Input: part model. Units: mm. Frame: model coordinates. A direction names the side the tool comes from. Round coordinates to 2 decimals unless told otherwise and drop trailing zeros. Loops run counter-clockwise (first coordinate to the right, second up) from the corner with the lowest first, then second, coordinate; pieces in that order, holes last.
1) Section D-D, the plane y = -22.5. Return loops of the section in (x, z), and give its area (3 significant figures).
2) Ray query, line 1 along X through (y, z) = (27, 0.55); line 2 along Y through (x, z) = (49, 0.75) (3 decimals); line 3 along Y through (x, z) = (10.5, 0.5). Return the intervals inside material, ascending.
3) Access query for faces 1 (the face through (26.94, 31.3, 0.78)), 2 (the face through (26.742, -37.615, 0.783)), 3 (the face through (-7.924, -11.766, 0.783)). Directions: +Z, -Z, +X, -X, +Y, -Y. A direction counts if a zero-diameter tool reaches every point of the face in a straight line with its end or side. Return the directions, or none.
4) Section A-A, the plane x = 25. Return loops of the section in (y, z).
5) Draft query along X for faces 4 (the face through (54.83, -43.89, 0.78)), 5 (the face through (-7.51, -29.71, 0.78)), 6 (the face through (2, -3, 1.588)). Return one class per face: pulls with the +X half, pulls with the -X half, needs draft (parallel to the pull), parting line crosses it, or undercut.
6) Section C-C, the plane z = 0.35. State how many separate pieces and enclosed holes the cut face has, and give its area (3 significant figures).
7) First-contact query: pin 1 (0.8 mm diameter, centred on x = 2, z = 0.5, fed in from -Y); pin 2 (0.5 mm diameter, centred on y = -40.5, z = 0.5, fed in from -X). Flat tips, straight axial feed; report the tip coordinate or a pass-through.
8) Section B-B, the plane x = -19. Return loops of the section in (y, z).
from build123d import *

# Parameters (mm, degrees)
F0_R     = 0.993004
F0_R_2   = 1.444011
F1_DEPTH = 1.5875


with BuildPart() as f1:
    # F0 (on Top) → F1 (new body)
    with BuildSketch(Plane.XY):
        with BuildLine():
            Line((-14.723098, 26.865108), (-29.863264, 35.613344))
            ThreePointArc((-29.863264, 35.613344), (-50.45729, 37.191393), (-38.937857, 20.047683))
            Line((-38.937857, 20.047683), (-12.721558, 4.9235))
            Line((-12.721558, 4.9235), (-11.685765, 4.128267))
            Line((-11.685765, 4.128267), (-10.891915, 3.094106))
            Line((-10.891915, 3.094106), (-10.393018, 1.886993))
            Line((-10.393018, 1.886993), (-10.222391, 0.594116))
            Line((-10.222391, 0.594116), (-10.220915, -7.038907))
            Line((-10.220915, -7.038907), (-10.393611, -8.33664))
            Line((-10.393611, -8.33664), (-10.893255, -9.537127))
            Line((-10.893255, -9.537127), (-11.691344, -10.573302))
            Line((-11.691344, -10.573302), (-12.744763, -11.375137))
            Line((-12.744763, -11.375137), (-38.796974, -26.421059))
            Line((-38.796974, -26.421059), (-38.877102, -26.468848))
            ThreePointArc((-38.877102, -26.468848), (-50.486605, -43.553232), (-29.883725, -42.077399))
            Line((-29.883725, -42.077399), (-14.723923, -33.307276))
            Line((-14.723923, -33.307276), (-13.889479, -32.979281))
            Line((-13.889479, -32.979281), (-12.998538, -32.911762))
            Line((-12.998538, -32.911762), (-12.125839, -33.111285))
            Line((-12.125839, -33.111285), (-11.353738, -33.556437))
            Line((-11.353738, -33.556437), (-10.745112, -34.212011))
            Line((-10.745112, -34.212011), (-10.356967, -35.016805))
            Line((-10.356967, -35.016805), (-10.221996, -35.901241))
            Line((-10.221996, -35.901241), (-10.221996, -46.300355))
            Line((-10.221996, -46.300355), (-10.074989, -47.230888))
            Line((-10.074989, -47.230888), (-9.656024, -48.045732))
            Line((-9.656024, -48.045732), (-8.990064, -48.723656))
            Line((-8.990064, -48.723656), (-8.144654, -49.150351))
            Line((-8.144654, -49.150351), (-7.219487, -49.297899))
            Line((-7.219487, -49.297899), (11.685274, -49.296624))
            Line((11.685274, -49.296624), (12.637615, -49.147114))
            Line((12.637615, -49.147114), (13.504221, -48.70079))
            Line((13.504221, -48.70079), (14.18661, -48.018399))
            Line((14.18661, -48.018399), (14.627374, -47.158636))
            Line((14.627374, -47.158636), (14.775819, -46.2091))
            Line((14.775819, -46.2091), (14.778971, -35.906233))
            Line((14.778971, -35.906233), (14.910567, -35.024933))
            Line((14.910567, -35.024933), (15.297383, -34.217406))
            Line((15.297383, -34.217406), (15.907513, -33.557428))
            Line((15.907513, -33.557428), (16.67915, -33.11279))
            Line((16.67915, -33.11279), (17.548487, -32.913399))
            Line((17.548487, -32.913399), (18.445739, -32.979199))
            Line((18.445739, -32.979199), (19.277777, -33.305883))
            Line((19.277777, -33.305883), (34.417649, -42.047282))
            ThreePointArc((34.417649, -42.047282), (55.015649, -43.582376), (43.457552, -26.463833))
            Line((43.457552, -26.463833), (17.281802, -11.366066))
            Line((17.281802, -11.366066), (16.244157, -10.573521))
            Line((16.244157, -10.573521), (15.449484, -9.535828))
            Line((15.449484, -9.535828), (14.94993, -8.331098))
            Line((14.94993, -8.331098), (14.780158, -7.041344))
            Line((14.780158, -7.041344), (14.780158, 0.595206))
            Line((14.780158, 0.595206), (14.94993, 1.885977))
            Line((14.94993, 1.885977), (15.448278, 3.091799))
            Line((15.448278, 3.091799), (16.244157, 4.133809))
            Line((16.244157, 4.133809), (17.277955, 4.923416))
            Line((17.277955, 4.923416), (43.350993, 19.979317))
            ThreePointArc((43.350993, 19.979317), (54.979423, 37.050162), (34.375281, 35.599827))
            Line((34.375281, 35.599827), (19.284697, 26.87011))
            Line((19.284697, 26.87011), (18.450038, 26.540194))
            Line((18.450038, 26.540194), (17.539247, 26.472519))
            Line((17.539247, 26.472519), (16.68203, 26.667085))
            Line((16.68203, 26.667085), (15.906996, 27.120017))
            Line((15.906996, 27.120017), (15.300046, 27.770561))
            Line((15.300046, 27.770561), (14.911061, 28.57871))
            Line((14.911061, 28.57871), (14.778835, 29.453185))
            Line((14.778835, 29.453185), (14.778835, 39.838884))
            Line((14.778835, 39.838884), (14.635858, 40.771108))
            Line((14.635858, 40.771108), (14.205475, 41.613926))
            Line((14.205475, 41.613926), (13.539729, 42.286281))
            Line((13.539729, 42.286281), (12.708107, 42.70209))
            Line((12.708107, 42.70209), (11.775819, 42.852354))
            Line((11.775819, 42.852354), (9.028588, 42.849436))
            Line((9.028588, 42.849436), (8.248972, 42.750109))
            Line((8.248972, 42.750109), (7.521199, 42.450108))
            Line((7.521199, 42.450108), (6.899957, 41.975875))
            Line((6.899957, 41.975875), (6.155663, 41.238896))
            Line((6.155663, 41.238896), (5.542562, 40.758778))
            Line((5.542562, 40.758778), (4.811539, 40.46033))
            Line((4.811539, 40.46033), (4.057043, 40.356379))
            Line((4.057043, 40.356379), (0.515512, 40.356379))
            Line((0.515512, 40.356379), (-0.251471, 40.45441))
            Line((-0.251471, 40.45441), (-0.987362, 40.755984))
            Line((-0.987362, 40.755984), (-1.601019, 41.228801))
            Line((-1.601019, 41.228801), (-2.333428, 41.96848))
            Line((-2.333428, 41.96848), (-2.958887, 42.448372))
            Line((-2.958887, 42.448372), (-3.688263, 42.751611))
            Line((-3.688263, 42.751611), (-4.465904, 42.852182))
            Line((-4.465904, 42.852182), (-7.223364, 42.850204))
            Line((-7.223364, 42.850204), (-8.143452, 42.702295))
            Line((-8.143452, 42.702295), (-8.975075, 42.283129))
            Line((-8.975075, 42.283129), (-9.64701, 41.617799))
            Line((-9.64701, 41.617799), (-10.078163, 40.777281))
            Line((-10.078163, 40.777281), (-10.221545, 39.848268))
            Line((-10.221545, 39.848268), (-10.221545, 29.468842))
            Line((-10.221545, 29.468842), (-10.356562, 28.594707))
            Line((-10.356562, 28.594707), (-10.741985, 27.769495))
            Line((-10.741985, 27.769495), (-11.349, 27.124543))
            Line((-11.349, 27.124543), (-12.121995, 26.674023))
            Line((-12.121995, 26.674023), (-12.989837, 26.475296))
            Line((-12.989837, 26.475296), (-13.889652, 26.536117))
            Line((-13.889652, 26.536117), (-14.723098, 26.865108))
        make_face()
        with Locations((-41.662121, -42.13991)):
            Circle(F0_R, mode=Mode.SUBTRACT)
        with Locations((-36.148938, -38.95656)):
            Circle(F0_R, mode=Mode.SUBTRACT)
        with Locations((-44.843597, -36.637466)):
            Circle(F0_R, mode=Mode.SUBTRACT)
        with Locations((-39.334769, -33.438058)):
            Circle(F0_R, mode=Mode.SUBTRACT)
        with Locations((-7.196873, -46.281218)):
            Circle(F0_R_2, mode=Mode.SUBTRACT)
        with Locations((-7.196873, -28.3006)):
            Circle(F0_R_2, mode=Mode.SUBTRACT)
        with Locations((-7.73577, -13.198138)):
            Circle(F0_R_2, mode=Mode.SUBTRACT)
        with Locations((11.686507, -46.199943)):
            Circle(F0_R_2, mode=Mode.SUBTRACT)
        with Locations((11.686507, -28.198998)):
            Circle(F0_R_2, mode=Mode.SUBTRACT)
        with Locations((40.701358, -38.95656)):
            Circle(F0_R, mode=Mode.SUBTRACT)
        with Locations((46.225792, -42.13991)):
            Circle(F0_R, mode=Mode.SUBTRACT)
        with Locations((49.40368, -36.637466)):
            Circle(F0_R, mode=Mode.SUBTRACT)
        with Locations((43.888332, -33.438058)):
            Circle(F0_R, mode=Mode.SUBTRACT)
        with Locations((12.255891, -13.198138)):
            Circle(F0_R_2, mode=Mode.SUBTRACT)
        with Locations((-7.730273, 6.771058)):
            Circle(F0_R_2, mode=Mode.SUBTRACT)
        with Locations((-39.334769, 27.009396)):
            Circle(F0_R, mode=Mode.SUBTRACT)
        with Locations((-44.843597, 30.177385)):
            Circle(F0_R, mode=Mode.SUBTRACT)
        with Locations((-41.662121, 35.696518)):
            Circle(F0_R, mode=Mode.SUBTRACT)
        with Locations((-36.148938, 32.520008)):
            Circle(F0_R, mode=Mode.SUBTRACT)
        with Locations((-7.234972, 21.847867)):
            Circle(F0_R_2, mode=Mode.SUBTRACT)
        with Locations((-7.196873, 39.856457)):
            Circle(F0_R_2, mode=Mode.SUBTRACT)
        with Locations((12.29907, 6.771058)):
            Circle(F0_R_2, mode=Mode.SUBTRACT)
        with Locations((11.772867, 21.847867)):
            Circle(F0_R_2, mode=Mode.SUBTRACT)
        with Locations((11.772867, 39.875787)):
            Circle(F0_R_2, mode=Mode.SUBTRACT)
        with Locations((43.888332, 27.009396)):
            Circle(F0_R, mode=Mode.SUBTRACT)
        with Locations((49.40368, 30.177385)):
            Circle(F0_R, mode=Mode.SUBTRACT)
        with Locations((40.705846, 32.520009)):
            Circle(F0_R, mode=Mode.SUBTRACT)
        with Locations((46.225792, 35.696518)):
            Circle(F0_R, mode=Mode.SUBTRACT)
    extrude(amount=F1_DEPTH)


solid = f1.part
Final values:
1. outline: (-32.01, 0) - (36.59, 0) - (36.59, 1.59) - (-32.01, 1.59) - close
1. area: 109 mm2
2. line 1: x = -51.14 to -40.33, -38.34 to -14.96, -11.56 to 16.11, 19.51 to 42.9, 44.88 to 55.66
2. line 2: y = -48.613 to -37.545, -35.73 to -27.034, 20.565 to 29.27, 31.085 to 42.1
2. line 3: y = -49.3 to -47.02, -45.38 to -29.02, -27.38 to 21.17, 22.53 to 39.19, 40.56 to 42.85
3. face 1: +Z, -Z, +Y
3. face 2: +Z, -Z, -Y
3. face 3: +Z, -Z
4. outline: (-36.61, 0) - (-15.82, 0) - (-15.82, 1.59) - (-36.61, 1.59) - close; (9.38, 0) - (30.18, 0) - (30.18, 1.59) - (9.38, 1.59) - close
5. face 4: undercut
5. face 5: undercut
5. face 6: needs draft
6. separate pieces: 1
6. enclosed holes: 28
6. area: 5,620 mm2
7. pin 1: stops at y = -49.3
7. pin 2: stops at x = -51.76
8. outline: (-35.78, 0) - (-14.99, 0) - (-14.99, 1.59) - (-35.78, 1.59) - close; (8.55, 0) - (29.34, 0) - (29.34, 1.59) - (8.55, 1.59) - close
